Read the model definition and answer for the solid it produces. Units are mm, in the model's axes. A direction names the side the tool comes from. Give positions to 0.01 mm unless a question says otherwise; leave off trailing zeros. Order: outer loops, then holes, each group sorted by start corner. A loop starts at its lowest first (then second) coordinate and runs counter-clockwise, first axis right, second up. Notation, with made-up numbers: (-36.5, 70.5) -> (-6.5, 70.5) arc R29 cw to (-6.5, 97.5) -> close; hole circle Ø1 at (-15.5, 20). An arc over 180 degrees is marked (long way). One line per item, written item: value. Start each with the question number.
from build123d import *

# Parameters (mm, degrees)
SKETCH_4_W      = 130
SKETCH_4_H      = 130
EXTRUDE_1_DEPTH = 200
SKETCH_5_W      = 130
SKETCH_5_H      = 130
EXTRUDE_2_DEPTH = 170


with BuildPart() as part:
    # 스케치4 → 보스-돌출1 (new body)
    with BuildSketch(Plane.XY):
        Rectangle(SKETCH_4_W, SKETCH_4_H)
        with BuildLine():
            Line((-49.749371855, 5), (-29.580398915, 5))
            ThreePointArc((-29.580398915, 5), (0, -30), (29.580398915, 5))
            Line((29.580398915, 5), (49.749371855, 5))
            ThreePointArc((49.749371855, 5), (0, -50), (-49.749371855, 5))
        make_face(mode=Mode.SUBTRACT)
    extrude(amount=EXTRUDE_1_DEPTH)

    # 스케치5 → 보스-돌출2 (add)
    with BuildSketch(Plane(origin=(0, 0, 0), x_dir=(-1, 0, 0), z_dir=(0, 0, -1))):
        Rectangle(SKETCH_5_W, SKETCH_5_H)
    extrude(amount=-EXTRUDE_2_DEPTH)


solid = part.part
Item 1: Find section A-A on z = 178. Write down the section's boundary in (x, y).
Item 2: Find section C-C on x = -40. Write down the section's boundary in (y, z).
Item 3: Find section B-B on y = -47.5. Write down the section's boundary in (x, z).
Item 4: For a pull along X with two mould halves and no side action, classify faces 1 (the flat face through (65, -1, 99)), 2 (the flat face through (-65, -1, 99)), 3 (the cylindrical face through (1.17, -49.986, 184.79)), 4 (the flat face through (-1, -65, 99)) as +X half, -X half, draft (parallel to the pull), parting line (faces both ways), or undercut.
Item 5: A flat-ended cylindrical pin translates along its axis: pin 1 (5 mm diameter, centred on x = 33.5, y = 14, fed in from -Z). Find the tip coordinate at first contact, or state that the pin passes through.
Item 6: A tool of negligible diameter and unlimited length cuts with its end or side. For faces 5 (the flat face through (40, 5, 185)), 6 (the flat face through (-1, 1, 0)), from which of +Z, -Z, +X, -X, +Y, -Y can it reach the whole face along a straight path? Write none if from no direction.
Item 7: Find section D-D on y = 0. Write down the section's boundary in (x, z).
Item 8: Find the intervals of material crossed by line 1 (X direction, y = 0, z = 190); line 2 (Y direction, x = -24.5, z = 176); line 3 (X direction, y = -16, z = 186), in increasing order. Write a range as from..to.
Checks:
1. outline: (-65, -65) -> (65, -65) -> (65, 65) -> (-65, 65) -> close; hole (-49.75, 5) arc R50 ccw (long way) to (49.75, 5) -> (29.58, 5) arc R30 cw (long way) to (-29.58, 5) -> close
2. outline: (-65, 0) -> (65, 0) -> (65, 200) -> (5, 200) -> (5, 170) -> (-30, 170) -> (-30, 200) -> (-65, 200) -> close
3. outline: (-65, 0) -> (65, 0) -> (65, 200) -> (15.61, 200) -> (15.61, 170) -> (-15.61, 170) -> (-15.61, 200) -> (-65, 200) -> close
4. face 1: +X half
4. face 2: -X half
4. face 3: undercut
4. face 4: draft
5. pin 1: z = 0
6. face 5: +Z
6. face 6: -Z, +X, -X, +Y, -Y
7. outline: (-65, 0) -> (65, 0) -> (65, 200) -> (50, 200) -> (50, 170) -> (30, 170) -> (30, 200) -> (-30, 200) -> (-30, 170) -> (-50, 170) -> (-50, 200) -> (-65, 200) -> close
8. line 1: -65..-50, -30..30, 50..65
8. line 2: -65..-43.59, -17.31..65
8. line 3: -65..-47.37, -25.38..25.38, 47.37..65
